Geometry: final body of the model. Coordinates: model frame, mm. Face numbers are marked on the shaded views. A direction names the side the tool comes from. Coordinates: 2 decimals unless noted, no trailing zeros. Loops run counter-clockwise (first coordinate to the right, second up) from the corner with the lowest first, then second, coordinate; pieces in that order, holes last. Notation, with made-up numbers: (74.25, 45) - (120.25, 45) arc R33 ccw to (120.25, 79) - close; hole circle Ø9 at (20.5, 27.5). An arc over 180 degrees is marked (long way). Return JSON: item names as keys, results as strings.
from build123d import *

# Parameters (mm, degrees)
BOSS_EXTRUDE1_DEPTH     = 82.55
SHELL1_START            = 6.35
SHELL1_DEPTH            = 69.85
SKETCH4_W               = 176.485735693
SKETCH4_H               = 90.097834431
CUT_EXTRUDE1_DEPTH      = 25.4
CUT_EXTRUDE2_DEPTH      = 113.522286681
CUT_EXTRUDE2_DEPTH_BACK = 113.522286681
SKETCH8_R               = 4.7625
SKETCH8_R_2             = 3.96875
CUT_EXTRUDE3_DEPTH      = 113.522286681


# Read off the part's stored shape, not the designer's step: Shell1
with BuildPart() as part:
    # Sketch1 → Boss-Extrude1 (new body)
    with BuildSketch(Plane.XY):
        Polygon((57.15, 0), (-57.15, 0), (-57.15, 6.35), (-32.186094587, 6.35), (-28.575, 47.625), (-22.200744032, 47.625), (-21.922967525, 50.8), (21.922967525, 50.8), (22.200744032, 47.625), (28.575, 47.625), (32.186094587, 6.35), (57.15, 6.35), align=None)
    extrude(amount=BOSS_EXTRUDE1_DEPTH)

    # Shell1 outline → Shell1 (cut)
    with BuildSketch(Plane.XY.offset(SHELL1_START)):
        Polygon((26.367391632, 0), (22.756297045, 41.275), (16.382041077, 41.275), (16.10426457, 44.45), (-16.10426457, 44.45), (-16.382041077, 41.275), (-22.756297045, 41.275), (-26.367391632, 0), align=None)
    extrude(amount=SHELL1_DEPTH, mode=Mode.SUBTRACT)

    # Sketch4 → Cut-Extrude1 (cut)
    with BuildSketch(Plane(origin=(0, 0, 0), x_dir=(1, 0, 0), z_dir=(0, 0.08715574274765504, -0.9961946980917459))):
        with Locations((12.432297096, -27.899571849)):
            Rectangle(SKETCH4_W, SKETCH4_H)
    cut_extrude1 = extrude(amount=CUT_EXTRUDE1_DEPTH, mode=Mode.SUBTRACT)

    # Sketch7 → Cut-Extrude2 (cut, two sides: drawn at the far end of the back side and taken through both)
    with BuildSketch(Plane(origin=(0, 0, 0), x_dir=(0, 0, -1), z_dir=(1, 0, 0)).offset(-CUT_EXTRUDE2_DEPTH_BACK)):
        Polygon((-4.1666476, 47.625), (-10.540903569, 47.625), (-10.818680076, 50.8), (-4.444424107, 50.8), align=None)
    extrude(amount=CUT_EXTRUDE2_DEPTH + CUT_EXTRUDE2_DEPTH_BACK, mode=Mode.SUBTRACT)

    # Mirror1: Cut-Extrude1 across plane
    add(cut_extrude1.mirror(Plane.XY.offset(41.275)), mode=Mode.SUBTRACT)

    # Sketch8 → Cut-Extrude3 (cut, through all)
    with BuildSketch(Plane(origin=(0, 50.8, 0), x_dir=(1, 0, 0), z_dir=(0, 1, 0))):
        with Locations(Location((0, -42.2666476, 0), (0, 0, 270))):
            Circle(SKETCH8_R)
        with Locations(Location((44.45, -56.594446987, 0), (0, 0, 270))):
            Circle(SKETCH8_R_2)
        with Locations(Location((-44.45, -56.594446987, 0), (0, 0, 270))):
            Circle(SKETCH8_R_2)
    extrude(amount=-CUT_EXTRUDE3_DEPTH, mode=Mode.SUBTRACT)


solid = part.part
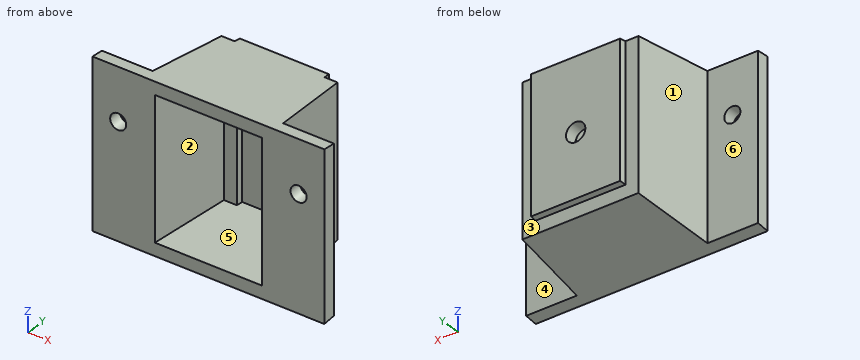
Item 1: Section query A-A, the plane x = 0. Return loops of the section in (y, z) (3 decimals), and give its area (3 significant figures).
Worked out:
{"outline": "(0, 0) - (47.625, 4.167) - (47.625, 10.541) - (50.8, 10.819) - (50.8, 37.504) - (44.45, 37.504) - (44.45, 6.35) - (0, 6.35) - close; (0, 76.2) - (44.45, 76.2) - (44.45, 47.029) - (50.8, 47.029) - (50.8, 78.106) - (0, 82.55) - close", "area": "782 mm^2"}
Item 2: Mould query, pull axis X, two halves, no side actions, for the marked faces 1, 2 and 3. Classes: +X half, -X half, draft (parallel to the pull), parting line (faces both ways), or undercut.
Worked out:
{"face 1": "-X half", "face 2": "undercut", "face 3": "draft"}
Item 3: Section query D-D, the plane z = 72.5. Return loops of the section in (x, y) (3 decimals), and give its area (3 significant figures).
Worked out:
{"outline": "(-57.15, 0) - (-26.367, 0) - (-22.756, 41.275) - (-16.382, 41.275) - (-16.104, 44.45) - (16.104, 44.45) - (16.382, 41.275) - (22.756, 41.275) - (26.367, 0) - (57.15, 0) - (57.15, 6.35) - (32.186, 6.35) - (28.575, 47.625) - (22.201, 47.625) - (21.923, 50.8) - (-21.923, 50.8) - (-22.201, 47.625) - (-28.575, 47.625) - (-32.186, 6.35) - (-57.15, 6.35) - close", "area": "1,240 mm^2"}
Item 4: Reachability of the marked faces 4, 5 and 6 from +Z, -Z, +X, -X, +Y, -Y: full face, straight path, thin tool, end or side. Return the list, or none.
Worked out:
{"face 4": "+Z, -Z, +X, +Y", "face 5": "-Y", "face 6": "+Z, -Z, -X, +Y"}
Item 5: Section query C-C, the plane x = 19. Return loops of the section in (y, z) (3 decimals).
Worked out:
{"outline": "(0, 0) - (47.625, 4.167) - (47.625, 10.541) - (50.8, 10.819) - (50.8, 78.106) - (0, 82.55) - (0, 76.2) - (41.275, 76.2) - (41.275, 6.35) - (0, 6.35) - close"}
Item 6: Section query B-B, the plane y = 21. Return loops of the section in (x, z), and give its area (3 significant figures).
Worked out:
{"outline": "(-30.9, 1.84) - (30.9, 1.84) - (30.9, 80.71) - (-30.9, 80.71) - close; hole (-24.53, 6.35) - (24.53, 6.35) - (24.53, 76.2) - (-24.53, 76.2) - close", "area": "1,450 mm^2"}
Item 7: Ray query, probe 1 along Z at (x, y) = (22.5, 47.5); probe 2 along Y at (x, z) = (39.5, 5.5); probe 3 along Y at (x, z) = (-20.5, 68) (3 decimals). Return the intervals inside material, ascending. Write a range as from..to.
Worked out:
{"probe 1": "4.16..78.39", "probe 2": "0..6.35", "probe 3": "41.275..50.8"}
Item 8: First-contact query: pin 1 Ø22 at (x, y) = (-7.5, 18) entering from -Z; pin 2 Ø5 at (y, z) = (23.5, 32.5) entering from +X; pin 3 Ø3 at (x, z) = (20.5, 56) entering from -Y (3 decimals). Flat tips, straight axial feed; report the tip coordinate or a pass-through.
Worked out:
{"pin 1": "z = 0.61", "pin 2": "x = 30.9", "pin 3": "y = 41.275"}
